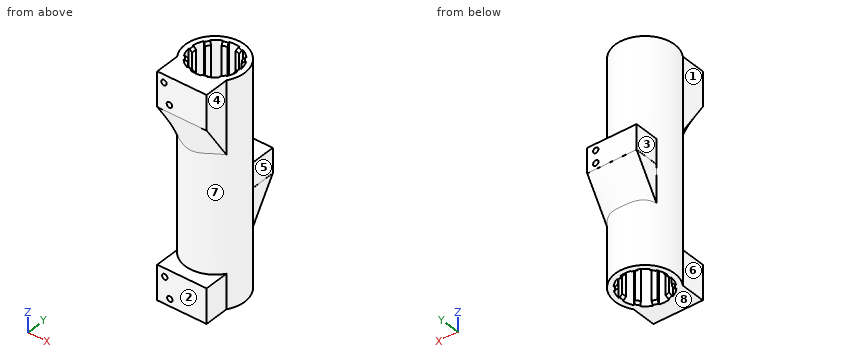
from build123d import *

# Parameters (mm, degrees)
CYLINDER_R     = 8.5
CYLINDER_DEPTH = 90
BOX_W          = 20
BOX_H          = 2
BOX_DEPTH      = 90
CHAMFER_SIZE   = 1
ARRAY_COUNT    = 5
SKETCH_R       = 12
SKETCH_R_2     = 9.92732
PAD_DEPTH      = 90
PAD001_DEPTH   = 14
PAD002_DEPTH   = 14
SKETCH005_R    = 1.1
HOLE_DEPTH     = 6
HOLE_TIPS_R    = 1.1
SKETCH006_R    = 1.1
HOLE001_DEPTH  = 7
HOLE001_TIPS_R = 1.1
PAD005_DEPTH   = 10
SKETCH034_R    = 1.1
HOLE002_DEPTH  = 7
HOLE002_TIPS_R = 1.1


with BuildPart() as cylinder:
    # Cylinder → Cylinder (new body)
    with BuildSketch(Plane.XY):
        Circle(CYLINDER_R)
    extrude(amount=CYLINDER_DEPTH)


with BuildPart() as main_circuit:
    # Box → Box (new body)
    with BuildSketch(Plane(origin=(-10, -1, 0), x_dir=(1, 0, 0), z_dir=(0, 0, 1))):
        with Locations((10, 1)):
            Rectangle(BOX_W, BOX_H)
    extrude(amount=BOX_DEPTH)

    # Cut: cut Cylinder
    add(cylinder.part, mode=Mode.SUBTRACT)

    # Chamfer
    chamfer_edges = [main_circuit.edges().sort_by_distance(p)[0] for p in [
        (-8.5, 0, 90),
        (-8.5, 0, 0),
        (8.48523, -0.50087, 0),
        (8.48523, 0.50087, 0),
        (8.48523, -0.50087, 90),
        (8.48523, 0.50087, 90),
    ]]
    chamfer(chamfer_edges, length=CHAMFER_SIZE)

    # Array: main_circuit ×5 about axis
    array_axis = Axis((0, 0, 0), (0, 0, 1))


with BuildPart() as main_circuit_1:
    add(main_circuit.part)
    for i in range(1, ARRAY_COUNT):
        add(main_circuit.part.rotate(array_axis, i * 360 / ARRAY_COUNT))

    # Sketch (on Face14 of Chamfer) → Pad (new body)
    with BuildSketch(Plane.XY.offset(90)):
        Circle(SKETCH_R)
        Circle(SKETCH_R_2, mode=Mode.SUBTRACT)
    extrude(amount=-PAD_DEPTH)

    # Sketch001 (on Face2 of Pad) → Pad001 (join)
    with BuildSketch(Plane.XY.offset(90)):
        with BuildLine():
            ThreePointArc((-10, -6.63325), (0, -12), (10, -6.63325))
            Line((10, -16.63325), (10, -6.63325))
            Line((-10, -16.63325), (10, -16.63325))
            Line((-10, -16.63325), (-10, -6.63325))
        make_face()
    extrude(amount=-PAD001_DEPTH)

    # Sketch003 (on Face2 of Pad) → Pad002 (join)
    with BuildSketch(Plane.XY):
        with BuildLine():
            ThreePointArc((-10, -6.63325), (0, -12), (10, -6.63325))
            Line((10, -16.63325), (10, -6.63325))
            Line((-10, -16.63325), (10, -16.63325))
            Line((-10, -16.63325), (-10, -6.63325))
        make_face()
    extrude(amount=PAD002_DEPTH)

    # Sketch005 → Hole (cut)
    with BuildSketch(Plane.XZ.offset(16.63325)):
        with Locations((-7.279865, 86.818527)):
            Circle(SKETCH005_R)
        with Locations((-5.058943, 79.102539)):
            Circle(SKETCH005_R)
    extrude(amount=-HOLE_DEPTH, mode=Mode.SUBTRACT)

    # Hole tips → Hole tip 1 section 0
    with BuildSketch(Plane.XZ.offset(10.63325), mode=Mode.PRIVATE) as hole_tip_1_s0:
        with Locations((-7.279865, 86.818527)):
            Circle(HOLE_TIPS_R)
    loft([hole_tip_1_s0.sketch, Vertex(-7.279865, -9.972303, 86.818527)], mode=Mode.SUBTRACT)

    # Hole tips → Hole tip 2 section 0
    with BuildSketch(Plane.XZ.offset(10.63325), mode=Mode.PRIVATE) as hole_tip_2_s0:
        with Locations((-5.058943, 79.102539)):
            Circle(HOLE_TIPS_R)
    loft([hole_tip_2_s0.sketch, Vertex(-5.058943, -9.972303, 79.102539)], mode=Mode.SUBTRACT)

    # Sketch006 (on Face31 of Hole) → Hole001 (cut)
    with BuildSketch(Plane.XZ.offset(16.63325)):
        with Locations((-6.949521, 10.656509)):
            Circle(SKETCH006_R)
        with Locations((-4.900103, 2.902877)):
            Circle(SKETCH006_R)
    extrude(amount=-HOLE001_DEPTH, mode=Mode.SUBTRACT)

    # Hole001 tips → Hole001 tip 1 section 0
    with BuildSketch(Plane.XZ.offset(9.63325), mode=Mode.PRIVATE) as hole001_tip_1_s0:
        with Locations((-6.949521, 10.656509)):
            Circle(HOLE001_TIPS_R)
    loft([hole001_tip_1_s0.sketch, Vertex(-6.949521, -8.972303, 10.656509)], mode=Mode.SUBTRACT)

    # Hole001 tips → Hole001 tip 2 section 0
    with BuildSketch(Plane.XZ.offset(9.63325), mode=Mode.PRIVATE) as hole001_tip_2_s0:
        with Locations((-4.900103, 2.902877)):
            Circle(HOLE001_TIPS_R)
    loft([hole001_tip_2_s0.sketch, Vertex(-4.900103, -8.972303, 2.902877)], mode=Mode.SUBTRACT)

    # Sketch002 (on Face2 of Pad) → Pad005 (join)
    with BuildSketch(Plane(origin=(0, 0, 50), x_dir=(-1, 0, 0), z_dir=(0, 0, 1))):
        with BuildLine():
            ThreePointArc((-10, -6.63325), (0, -12), (10, -6.63325))
            Line((10, -16.63325), (10, -6.63325))
            Line((-10, -16.63325), (10, -16.63325))
            Line((-10, -16.63325), (-10, -6.63325))
        make_face()
    extrude(amount=-PAD005_DEPTH)

    # Sketch008 (on Face12 of Pad005) → AdditiveLoft section 0
    with BuildSketch(Plane(origin=(-10, 0, 0), x_dir=(0, -1, 0), z_dir=(-1, 0, 0))):
        Polygon((-16.636869, 39.970264), (-6.629684, 39.970264), (-6.629684, 24.694645), align=None)
    # Sketch009 (on Face12 of Pad005) → AdditiveLoft section 1
    with BuildSketch(Plane(origin=(0, 0, 0), x_dir=(0, -1, 0), z_dir=(-1, 0, 0))):
        Polygon((-16.637928, 39.961704), (-11.980004, 39.961704), (-11.980004, 24.806454), align=None)
    # Sketch010 (on Face12 of Pad005) → AdditiveLoft section 2
    with BuildSketch(Plane(origin=(10, 0, 0), x_dir=(0, -1, 0), z_dir=(-1, 0, 0))):
        Polygon((-16.634577, 39.974693), (-6.626975, 39.974693), (-6.626975, 24.656189), align=None)
    loft()

    # Sketch011 (on Face9 of AdditiveLoft) → AdditiveLoft001 section 0
    with BuildSketch(Plane.YZ.offset(10)):
        Polygon((-16.623207, 76.040215), (-6.641595, 76.040215), (-6.641595, 60.720215), align=None)
    # Sketch013 (on Face9 of AdditiveLoft) → AdditiveLoft001 section 1
    with BuildSketch(Plane.YZ):
        Polygon((-16.617746, 76.00518), (-11.950053, 76.00518), (-11.950053, 60.68518), align=None)
    # Sketch012 (on Face9 of AdditiveLoft) → AdditiveLoft001 section 2
    with BuildSketch(Plane.YZ.offset(-10)):
        Polygon((-16.629562, 76.014336), (-6.656822, 76.014336), (-6.656822, 60.706722), align=None)
    loft()

    # Sketch034 → Hole002 (cut)
    with BuildSketch(Plane(origin=(0, 16.63325, 0), x_dir=(-1, 0, 0), z_dir=(0, 1, 0))):
        with Locations((-6.56569, 47.399509)):
            Circle(SKETCH034_R)
        with Locations((-6.541382, 42.386913)):
            Circle(SKETCH034_R)
    extrude(amount=-HOLE002_DEPTH, mode=Mode.SUBTRACT)

    # Hole002 tips → Hole002 tip 1 section 0
    with BuildSketch(Plane(origin=(0, 9.63325, 0), x_dir=(-1, 0, 0), z_dir=(0, 1, 0)), mode=Mode.PRIVATE) as hole002_tip_1_s0:
        with Locations((-6.56569, 47.399509)):
            Circle(HOLE002_TIPS_R)
    loft([hole002_tip_1_s0.sketch, Vertex(6.56569, 8.972303, 47.399509)], mode=Mode.SUBTRACT)

    # Hole002 tips → Hole002 tip 2 section 0
    with BuildSketch(Plane(origin=(0, 9.63325, 0), x_dir=(-1, 0, 0), z_dir=(0, 1, 0)), mode=Mode.PRIVATE) as hole002_tip_2_s0:
        with Locations((-6.541382, 42.386913)):
            Circle(HOLE002_TIPS_R)
    loft([hole002_tip_2_s0.sketch, Vertex(6.541382, 8.972303, 42.386913)], mode=Mode.SUBTRACT)


solid = main_circuit_1.part
Design review of the part built by this model. Coordinates are the model's own, in mm. Face numbers are marked on the shaded views. A direction names the side the tool comes from. Coordinates: 2 decimals unless noted, no trailing zeros. Order: outer loops, then holes, each group sorted by start corner. A loop starts at its lowest first (then second) coordinate and runs counter-clockwise, first axis right, second up. Notation, with made-up numbers: (43.5, 46) -> (69.5, 46) arc R30 cw to (69.5, 72) -> close; hole circle Ø11 at (52.25, 42). An arc over 180 degrees is marked (long way). Use one line per item in the form item = value. Start each with the question number.
(1) For probe 1 along Y at (x, z) = (-0.5, 47.5); probe 2 along X at (y, z) = (-9, 54.5); probe 3 along X at (y, z) = (-4.5, 22), list the stretches that pass through material, from the lowest coordinate up.
(2) Add section A-A on y = 0. State the section outline as (x, z) points.
(3) The part is to be moulded in two halves that separate along Z. For the marked faces 6, 7 and 8, say which applies: +Z half, -Z half, draft (parallel to the pull), parting line (faces both ways), or undercut.
(4) For the marked faces 1, 2, 3, 4 and 5, list the 3-axis set-ups (+Z, -Z, +X, -X, +Y, -Y) from which the entire face can be reached by the end or side of a thin tool; tool diameter is ignored.
(5) Insertion check: pin 1 (1.1 mm diameter, centred on x = 9, z = 34, fed in from -Y); pin 2 (4 mm diameter, centred on x = 8.5, z = 20, fed in from +Y); pin 3 (2 mm diameter, centred on x = -5.06, z = 79.1, fed in from -Y); pin 4 (3 mm diameter, centred on x = -6.5, y = 2, fed in from -Z). Each pin has a flat end and moves straight along its axis. Give the tip position at first contact, or say it passes through.
(6) Add section B-B on y = 13.5. Give the number of separate pieces and of enclosed holes in the cut face, plus the area to 3 significant figures.
Answer block:
q1.probe_1 = -11.99 to -9.91, 9.91 to 16.63
q1.probe_2 = -7.94 to -4.19, -3.98 to -1.87, 1.87 to 3.98, 4.19 to 7.94
q1.probe_3 = -11.12 to -8.85, -7.9 to -7.21, 7.21 to 7.9, 8.85 to 11.12
q2.outline = (-12, 0) -> (-9.5, 0) -> (-8.5, 1) -> (-8.5, 89) -> (-9.5, 90) -> (-12, 90) -> close; (8.5, 1) -> (9.5, 0) -> (12, 0) -> (12, 90) -> (9.5, 90) -> (8.5, 89) -> close
q3.face_6 = draft
q3.face_7 = undercut
q3.face_8 = -Z half
q4.face_1 = +Z, -Z, -X, -Y
q4.face_2 = +Z, -Z, +X, -X, -Y
q4.face_3 = +Z, -Z, -X, +Y
q4.face_4 = +Z, -Z, +X, -Y
q4.face_5 = +Z, -Z, +X, +Y
q5.pin_1 = -8.52
q5.pin_2 = 10.09
q5.pin_3 = -10.57
q5.pin_4 = through
q6.separate_pieces = 2
q6.enclosed_holes = 2
q6.area = 349 mm²
